from build123d import *

# Parameters (mm, degrees)
SKETCH1_R               = 7.5
BOSS_EXTRUDE1_DEPTH     = 300
SKETCH3_W               = 5
SKETCH3_H               = 30
BOSS_EXTRUDE2_DEPTH     = 300
SKETCH4_W               = 70
SKETCH4_H               = 5
BOSS_EXTRUDE3_DEPTH     = 300
CUT_EXTRUDE1_DEPTH      = 305.353823699
CUT_EXTRUDE1_DEPTH_BACK = 305.353823699
SKETCH6_R               = 4


with BuildPart() as part:
    # Sketch1 → Boss-Extrude1 (new body)
    with BuildSketch(Plane.XY):
        Circle(SKETCH1_R)
    extrude(amount=BOSS_EXTRUDE1_DEPTH)

    # Sketch3 → Boss-Extrude2 (add)
    with BuildSketch(Plane.XY.offset(300)):
        with Locations((0, 15)):
            Rectangle(SKETCH3_W, SKETCH3_H)
    extrude(amount=-BOSS_EXTRUDE2_DEPTH)

    # Sketch4 → Boss-Extrude3 (add)
    with BuildSketch(Plane.XY.offset(300)):
        with Locations((0, 27.5)):
            Rectangle(SKETCH4_W, SKETCH4_H)
    extrude(amount=-BOSS_EXTRUDE3_DEPTH)

    # Sketch6 → Cut-Extrude1 (cut, two sides: drawn at the far end of the back side and taken through both)
    with BuildSketch(Plane(origin=(0, 30, 0), x_dir=(1, 0, 0), z_dir=(0, 1, 0)).offset(-CUT_EXTRUDE1_DEPTH_BACK)):
        with Locations(Location((-25, -5, 0), (0, 0, 270))):
            Circle(SKETCH6_R)
        with Locations(Location((25, -5, 0), (0, 0, 270))):
            Circle(SKETCH6_R)
        with Locations(Location((25, -295, 0), (0, 0, 270))):
            Circle(SKETCH6_R)
        with Locations(Location((-25, -295, 0), (0, 0, 270))):
            Circle(SKETCH6_R)
    extrude(amount=CUT_EXTRUDE1_DEPTH + CUT_EXTRUDE1_DEPTH_BACK, mode=Mode.SUBTRACT)


solid = part.part
Source: CAD feature listing. Evaluate the final solid. Frame: model axes, mm. A direction names the side the tool comes from. Coordinates: 2 decimals unless noted, no trailing zeros. Order: outer loops, then holes, each group sorted by start corner. A loop starts at its lowest first (then second) coordinate and runs counter-clockwise, first axis right, second up.
Item 1: Cut plane C-C (y = 0). Return loops of the section in (x, z), plus the area to 3 significant figures.
Output values:
outline: (-7.5, 0) - (7.5, 0) - (7.5, 300) - (-7.5, 300) - close
area: 4,500 mm2
Item 2: Set-up query: faces 1 (the face through (2.5, 16, 152)), 2 (the face through (0, 20, 300)), 3 (the face through (-2.5, 16, 152)). Return all of +Z, -Z, +X, -X, +Y, -Y with unobstructed straight access to the full face (end or side cutting, diameter ignored); none if empty.
Output values:
face 1: +Z, -Z, +X
face 2: +Z, +X, -X, +Y, -Y
face 3: +Z, -Z, -X
Item 3: Pull-direction query (X, two-part tool) for faces 4 (the face through (0, 20, 0)), 5 (the face through (25, 27, 291)), 6 (the face through (35, 27, 152)), 7 (the face through (28.966, 27.465, 4.479)); classes: pulls with the +X half, pulls with the -X half, needs draft (parallel to the pull), parting line crosses it, or undercut.
Output values:
face 4: needs draft
face 5: undercut
face 6: pulls with the +X half
face 7: undercut
Item 4: Cut plane B-B (z = 145). Return loops of the section in (x, y).
Output values:
outline: (-35, 25) - (-2.5, 25) - (-2.5, 7.07) arc R7.5 ccw (long way) to (2.5, 7.07) - (2.5, 25) - (35, 25) - (35, 30) - (-35, 30) - close
Item 5: Material intervals for line 1 (Z direction, x = -25, y = 28.9); line 2 (X direction, y = 28, z = 295); line 3 (Y direction, x = -27.5, z = 243), sorted ascending.
Output values:
line 1: z = 0 to 1, 9 to 291, 299 to 300
line 2: x = -35 to -29, -21 to 21, 29 to 35
line 3: y = 25 to 30
Item 6: Cut plane A-A (x = 25). Return loops of the section in (y, z), plus the area to 3 significant figures.
Output values:
outline: (25, 0) - (30, 0) - (30, 1) - (25, 1) - close; (25, 9) - (30, 9) - (30, 291) - (25, 291) - close; (25, 299) - (30, 299) - (30, 300) - (25, 300) - close
area: 1,420 mm2
Item 7: Cut plane D-D (y = 14). Return loops of the section in (x, z).
Output values:
outline: (-2.5, 0) - (2.5, 0) - (2.5, 300) - (-2.5, 300) - close
Item 8: First-contact query: P1, Ø4, axis at x = -9.5, y = 2, coming from the +Z side; P2, Ø5, axis at y = 0, z = 131, coming from the +X side; P3, Ø4, axis at y = 17.5, z = 98.5, coming from the -X side; P4, Ø19.5, axis at y = 14.5, z = 179, coming from the +X side. Flat tips, straight axial feed; report the tip coordinate or a pass-through.
Output values:
P1: passes through
P2: stops at x = 7.5
P3: stops at x = -2.5
P4: stops at x = 5.8
